Build history of the part. All positions in model axes, mm. A direction names the side the tool comes from. Give positions to 0.01 mm unless a question says otherwise; leave off trailing zeros. Order: outer loops, then holes, each group sorted by start corner. A loop starts at its lowest first (then second) coordinate and runs counter-clockwise, first axis right, second up. Notation, with made-up numbers: (9.5, 47) -> (43.5, 47) arc R16 ccw to (43.5, 75) -> close; hole circle Ø1 at (-10, 39). An arc over 180 degrees is marked (long way). Write item = value, one per line. Start each with the question number.
from build123d import *

# Parameters (mm, degrees)
BOSS_EXTRUDE1_DEPTH = 3
SKETCH2_R           = 1.5
CUT_EXTRUDE1_DEPTH  = 10
FILLET1_R           = 3
FILLET2_R           = 2


with BuildPart() as part:
    # Sketch1 → Boss-Extrude1 (new, symmetric)
    with BuildSketch(Plane(origin=(0, 0, 0), x_dir=(1, 0, 0), z_dir=(0, 1, 0))):
        with BuildLine():
            Line((6, 0), (6, -12.956788481))
            Line((6, -12.956788481), (-5, -24))
            Line((-5, -24), (-5, -34))
            Line((-5, -34), (10, -34))
            Line((10, -34), (10, 16))
            Line((10, 16), (-5, 16))
            Line((-5, 16), (-10.559794957, 5.700064076))
            ThreePointArc((-10.559794957, 5.700064076), (-11.634378786, 2.939596955), (-12, 0))
            Line((-12, 0), (-12, -8))
            Line((-12, -8), (-6, -8))
            Line((-6, -8), (-6, 0))
            ThreePointArc((-6, 0), (0, 6), (6, 0))
        make_face()
    extrude(amount=BOSS_EXTRUDE1_DEPTH, both=True)

    # Sketch2 → Cut-Extrude1 (cut)
    with BuildSketch(Plane(origin=(10, 0, 0), x_dir=(0, 0, -1), z_dir=(1, 0, 0))):
        with Locations((-28.5, 0)):
            Circle(SKETCH2_R)
        with Locations((10.5, 0)):
            Circle(SKETCH2_R)
    extrude(amount=-CUT_EXTRUDE1_DEPTH, mode=Mode.SUBTRACT)

    # Fillet1
    fillet1_edges = [part.edges().sort_by_distance(p)[0] for p in [
        (-5, 0, -16),
        (-5, 0, 34),
        (-5, 0, 24),
        (6, 0, 12.956788481),
    ]]
    fillet(fillet1_edges, radius=FILLET1_R)

    # Fillet2
    fillet2_edges = [part.edges().sort_by_distance(p)[0] for p in [
        (-6, 0, 8),
        (-12, 0, 8),
    ]]
    fillet(fillet2_edges, radius=FILLET2_R)


solid = part.part
(1) 3-axis set-ups, long thin cutter, end or side, ignore diameter. For faces 1 (the face through (-9, 0, 8)), 2 (the face through (5.8, 0, 12.8)), 3 (the face through (5, 0, -9)): which of +Z, -Z, +X, -X, +Y, -Y reach the whole face in a straight line?
(2) Cut at D-D, the plane z = -10.5. Give the cut face in (x, y).
(3) Flat gauge pins, fed straight in: P1, Ø3.5, axis at y = 0, z = 28.5, coming from the -X side; P2, Ø1.5, axis at y = -0.5, z = 28.5, coming from the +X side; P3, Ø2.5, axis at y = 0, z = -10.5, coming from the -X side. Where does each tip first touch, or does it go through?
(4) Mould opens along Z. For faces 4 (the face through (0, 0, 29)), 5 (the face through (10, 0, 9)), 6 (the face through (-4.14, 0.04, 33.1)), 7 (the face through (-4.728, 0.042, -15.588)) say: released by +Z, released by -Z, zero draft, split by the parting line, or undercut.
(5) Wall check: line 1 (Y direction, x = 3.75, z = 28.5); line 2 (Z direction, x = 5, y = 1.3); line 3 (X direction, y = -2.25, z = 27.5). Give the ranges that are in metal, low to high. Write a range as [from, to].
(6) Cut at A-A, the plane z = 3. Give the cut face in (x, y).
(7) Cut at C-C, the plane x = -1.5. Give the cut face in (y, z), plus the area to 3 significant figures.
(8) Cut at B-B, the plane y = 0. Give the cut face in (x, z).
Results:
q1.face_1 = +Z, -X, +Y, -Y
q1.face_2 = -X, +Y, -Y
q1.face_3 = +X
q2.outline = (-7.97, -3) -> (10, -3) -> (10, -1.5) -> (0, -1.5) -> (0, 1.5) -> (10, 1.5) -> (10, 3) -> (-7.97, 3) -> close
q3.P1 = -5
q3.P2 = 0
q3.P3 = -8.64
q4.face_4 = undercut
q4.face_5 = zero draft
q4.face_6 = released by +Z
q4.face_7 = released by -Z
q5.line_1 = [-3, -1.5], [1.5, 3]
q5.line_2 = [-16, -11.25], [-9.75, -3.32], [13.96, 27.75], [29.25, 34]
q5.line_3 = [-5, 10]
q6.outline = (-12, -3) -> (-6, -3) -> (-6, 3) -> (-12, 3) -> close; (6, -3) -> (10, -3) -> (10, 3) -> (6, 3) -> close
q7.outline = (-3, -16) -> (3, -16) -> (3, -5.81) -> (-3, -5.81) -> close; (-3, 20.49) -> (3, 20.49) -> (3, 34) -> (-3, 34) -> close
q7.area = 142 mm2
q8.outline = (-12, 0) arc R12 ccw to (-10.56, -5.7) -> (-5.85, -14.43) arc R3 ccw to (-3.21, -16) -> (10, -16) -> (10, -12) -> (0, -12) -> (0, -9) -> (10, -9) -> (10, 27) -> (0, 27) -> (0, 30) -> (10, 30) -> (10, 34) -> (-2, 34) arc R3 ccw to (-5, 31) -> (-5, 25.24) arc R3 ccw to (-4.13, 23.12) -> (5.13, 13.83) arc R3 cw to (6, 11.72) -> (6, 0) arc R6 cw to (-6, 0) -> (-6, 6) arc R2 ccw to (-8, 8) -> (-10, 8) arc R2 ccw to (-12, 6) -> close
